Check sheet for the modelled part. Datum: model origin and axes. Units: mm. Face numbers are marked on the shaded views. A direction names the side the tool comes from. Give positions to 0.01 mm unless a question says otherwise; leave off trailing zeros. Write each loop counter-clockwise with the first axis right and the second up, starting at its lowest first coordinate (ties: lowest second). Pieces come first, ordered by that corner, then holes. Notation, with made-up numbers: (-16.75, 60) -> (13.25, 60) arc R9 cw to (13.25, 71) -> close; hole circle Ø10 at (47, -32). An arc over 180 degrees is marked (long way). Use a Markdown table: item, result. Add a question column.
1. Cross-section at C-C (y = -4.5). Enter the section's corners in (x, z) (3 decimals), then the cut area to 3 significant figures.
2. Release check for a two-part mould opening along X. For the marked faces 1, 2 and 3 record: released by +X, released by -X, zero draft, split by the parting line, or undercut.
3. Cross-section at A-A (x = 6). Enter the section's corners in (y, z), then the cut area to 3 significant figures.
4. Gauge pin test, flat end, axial feed: P1, Ø3.5, axis at x = 8, z = -12.5, coming from the +Y side. Record the tip position at first contact, or that the pin passes through.
5. Scan lines: probe 1 along X at (y, z) = (-0.75, -7); probe 2 along Y at (x, z) = (11.5, -6.5); probe 3 along Y at (x, z) = (8.5, -5.5). Record each from-to range of solid material in increasing order. Write a range as [from, to].
6. Cross-section at D-D (x = 1.5). Enter the section's corners in (y, z).
7. Cross-section at B-B (z = -3). Enter the section's corners in (x, y), then the cut area to 3 significant figures.
8. Set-up check for the marked faces 4, 5 and 6: record each of +Z, -Z, +X, -X, +Y, -Y from which the full face is reachable in a straight line by a thin tool's end or side.
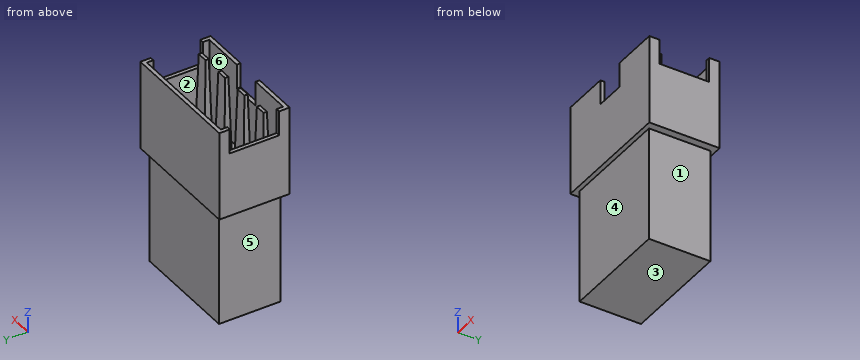
from build123d import *

# Parameters (mm, degrees)
SKETCH1_W           = 12.53
SKETCH1_H           = 7.1
BOSS_EXTRUDE1_DEPTH = 9
SKETCH2_W           = 11.73
SKETCH2_H           = 6.3
CUT_EXTRUDE1_DEPTH  = 8.5
SKETCH4_W           = 0.4
SKETCH4_H           = 5
SKETCH4_W_2         = 0.402982855
SKETCH4_W_3         = 3
SKETCH4_H_2         = 0.4
CUT_EXTRUDE3_DEPTH  = 2.5
SKETCH5_W           = 1.5
SKETCH5_H           = 0.750222952
BOSS_EXTRUDE4_DEPTH = 8
BOSS_EXTRUDE4_TAPER = 1.5
SKETCH8_W           = 11
SKETCH8_H           = 6.192617785
BOSS_EXTRUDE5_DEPTH = 11.5


with BuildPart() as part:
    # Sketch1 → Boss-Extrude1 (new body)
    with BuildSketch(Plane.XY):
        with Locations((6.265, -3.55)):
            Rectangle(SKETCH1_W, SKETCH1_H)
    extrude(amount=-BOSS_EXTRUDE1_DEPTH)

    # Sketch2 → Cut-Extrude1 (cut)
    with BuildSketch(Plane.XY):
        with Locations((6.265, -3.55)):
            Rectangle(SKETCH2_W, SKETCH2_H)
    extrude(amount=-CUT_EXTRUDE1_DEPTH, mode=Mode.SUBTRACT)

    # Sketch4 → Cut-Extrude3 (cut)
    with BuildSketch(Plane.XY):
        with Locations((0.2, -3.55)):
            Rectangle(SKETCH4_W, SKETCH4_H)
        with Locations((12.328508573, -3.55)):
            Rectangle(SKETCH4_W_2, SKETCH4_H)
        with Locations((6.265, -6.9)):
            Rectangle(SKETCH4_W_3, SKETCH4_H_2)
    extrude(amount=-CUT_EXTRUDE3_DEPTH, mode=Mode.SUBTRACT)

    # Sketch5 → Boss-Extrude4 (add)
    with BuildSketch(Plane.XY.offset(-8.5)):
        with Locations((1.65, -5.348826407)):
            Rectangle(SKETCH5_W, SKETCH5_H)
        with Locations((4.71, -5.348826407)):
            Rectangle(SKETCH5_W, SKETCH5_H)
        with Locations((7.77, -5.348826407)):
            Rectangle(SKETCH5_W, SKETCH5_H)
        with Locations((10.88, -5.348826407)):
            Rectangle(SKETCH5_W, SKETCH5_H)
    extrude(amount=BOSS_EXTRUDE4_DEPTH, taper=BOSS_EXTRUDE4_TAPER)

    # Sketch8 → Boss-Extrude5 (add)
    with BuildSketch(Plane(origin=(0, 0, -9), x_dir=(-1, 0, 0), z_dir=(0, 0, -1))):
        with Locations((-6.265, -3.552075665)):
            Rectangle(SKETCH8_W, SKETCH8_H)
    extrude(amount=BOSS_EXTRUDE5_DEPTH)


solid = part.part
Worked answers:
| question | item | result |
|---|---|---|
| 1 | outline | (0, -9) -> (0.765, -9) -> (0.765, -20.5) -> (11.765, -20.5) -> (11.765, -9) -> (12.53, -9) -> (12.53, -2.5) -> (12.13, -2.5) -> (12.13, -8.5) -> (0.4, -8.5) -> (0.4, -2.5) -> (0, -2.5) -> close |
| 1 | area | 138 mm² |
| 2 | face 1 | released by +X |
| 2 | face 2 | undercut |
| 2 | face 3 | zero draft |
| 3 | outline | (-7.1, -9) -> (-6.65, -9) -> (-6.65, -20.5) -> (-0.46, -20.5) -> (-0.46, -9) -> (0, -9) -> (0, 0) -> (-0.4, 0) -> (-0.4, -8.5) -> (-6.7, -8.5) -> (-6.7, -2.5) -> (-7.1, -2.5) -> close |
| 3 | area | 80.6 mm² |
| 4 | P1 | stops at y = -0.46 |
| 5 | probe 1 | x = [0, 0.4], [12.13, 12.53] |
| 5 | probe 2 | y = [-7.1, -6.7], [-5.67, -5.03], [-0.4, 0] |
| 5 | probe 3 | y = [-7.1, -6.7], [-0.4, 0] |
| 6 | outline | (-7.1, -9) -> (-6.65, -9) -> (-6.65, -20.5) -> (-0.46, -20.5) -> (-0.46, -9) -> (0, -9) -> (0, 0) -> (-0.4, 0) -> (-0.4, -8.5) -> (-4.97, -8.5) -> (-5.18, -0.5) -> (-5.51, -0.5) -> (-5.72, -8.5) -> (-6.7, -8.5) -> (-6.7, 0) -> (-7.1, 0) -> close |
| 7 | outline | (0, -7.1) -> (12.53, -7.1) -> (12.53, 0) -> (0, 0) -> close; (1.04, -5.58) -> (2.26, -5.58) -> (2.26, -5.12) -> (1.04, -5.12) -> close; (4.1, -5.58) -> (5.32, -5.58) -> (5.32, -5.12) -> (4.1, -5.12) -> close; (7.16, -5.58) -> (8.38, -5.58) -> (8.38, -5.12) -> (7.16, -5.12) -> close; (10.27, -5.58) -> (11.49, -5.58) -> (11.49, -5.12) -> (10.27, -5.12) -> close; hole (0.4, -6.7) -> (12.13, -6.7) -> (12.13, -0.4) -> (0.4, -0.4) -> close |
| 7 | area | 17.3 mm² |
| 8 | face 4 | -Z, +X, -X, -Y |
| 8 | face 5 | -Z, -X, +Y, -Y |
| 8 | face 6 | +Z |
